Input: part model. Units: mm. Frame: model coordinates. Face numbers are marked on the shaded views. A direction names the side the tool comes from. Coordinates: 2 decimals unless noted, no trailing zeros. Write each loop counter-clockwise with the first axis right and the second up, starting at its lowest first coordinate (ties: lowest second). Pieces come first, ordered by that corner, then holes. Notation, with made-up numbers: (66.25, -38) -> (115.25, -38) arc R10 cw to (115.25, -32) -> close; hole circle Ø6 at (-18, 1). An arc over 180 degrees is marked (long way). Use one line per item in the form item = value. Start each with the question number.
(1) First-contact query: pin 1 (4 mm diameter, centred on x = 6.5, y = -5, fed in from -Z); pin 2 (8.5 mm diameter, centred on x = 7, y = -4, fed in from +Z). Flat tips, straight axial feed; report the tip coordinate or a pass-through.
(2) Cut plane A-A on y = 53.5. Return the cut outline in (x, z).
(3) Cut plane B-B on z = 18. Return the cut outline in (x, y), plus the area to 3 significant figures.
(4) Set-up query: the marked faces 4 and 5. Return all of +Z, -Z, +X, -X, +Y, -Y with unobstructed straight access to the full face (end or side cutting, diameter ignored); none if empty.
(5) Cut plane C-C on x = -27.5. Return the cut outline in (y, z), plus the area to 3 significant figures.
(6) Pull-direction query (Y, two-part tool) for the marked faces 1, 2 and 3; classes: released by +Y, released by -Y, zero draft, split by the parting line, or undercut.
(7) Cut plane D-D on z = 30.5. Return the cut outline in (x, y), plus the area to 3 significant figures.
(8) Ray query, line 1 along X through (y, z) = (20, -16.5); line 2 along Y through (x, z) = (-21.5, -30); line 3 along X through (y, z) = (64, 27.5). Return the intervals inside material, ascending.
```python
from build123d import *

# Parameters (mm, degrees)
SALIENTE_EXTRUIR1_DEPTH = 50
CORTAR_EXTRUIR1_DEPTH   = 10


with BuildPart() as part:
    # Croquis1 → Saliente-Extruir1 (new, symmetric)
    with BuildSketch(Plane.XY):
        Polygon((-50, 0), (50, 0), (50, 60), (20, 60), (20, 67.9375), (57.9375, 67.9375), (57.9375, -7.9375), (-57.9375, -7.9375), (-57.9375, 67.9375), (-20, 67.9375), (-20, 60), (-50, 60), align=None)
    extrude(amount=SALIENTE_EXTRUIR1_DEPTH, both=True)

    # Croquis2 → Cortar-Extruir1 (cut)
    with BuildSketch(Plane.XZ.offset(7.9375)):
        Polygon((-28.867513459, -50), (28.867513459, -50), (14.43375673, -25), (-14.43375673, -25), align=None)
        Polygon((-28.867513459, 50), (28.867513459, 50), (14.43375673, 25), (-14.43375673, 25), align=None)
    extrude(amount=-CORTAR_EXTRUIR1_DEPTH, mode=Mode.SUBTRACT)


solid = part.part
```
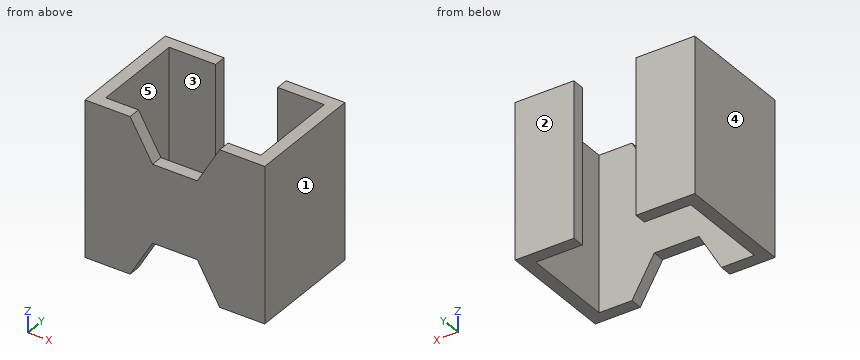
Values:
q1.pin_1 = -25
q1.pin_2 = 25
q2.outline = (-57.94, -50) -> (-50, -50) -> (-50, 50) -> (-57.94, 50) -> close; (50, -50) -> (57.94, -50) -> (57.94, 50) -> (50, 50) -> close
q3.outline = (-57.94, -7.94) -> (57.94, -7.94) -> (57.94, 67.94) -> (20, 67.94) -> (20, 60) -> (50, 60) -> (50, 0) -> (-50, 0) -> (-50, 60) -> (-20, 60) -> (-20, 67.94) -> (-57.94, 67.94) -> close
q3.area = 2,470 mm2
q4.face_4 = +Z, -Z, -X, +Y, -Y
q4.face_5 = +Z, -Z
q5.outline = (-7.94, -47.63) -> (0, -47.63) -> (0, 47.63) -> (-7.94, 47.63) -> close; (60, -50) -> (67.94, -50) -> (67.94, 50) -> (60, 50) -> close
q5.area = 1,550 mm2
q6.face_1 = zero draft
q6.face_2 = released by +Y
q6.face_3 = undercut
q7.outline = (-57.94, -7.94) -> (-17.61, -7.94) -> (-17.61, 0) -> (-50, 0) -> (-50, 60) -> (-20, 60) -> (-20, 67.94) -> (-57.94, 67.94) -> close; (17.61, -7.94) -> (57.94, -7.94) -> (57.94, 67.94) -> (20, 67.94) -> (20, 60) -> (50, 60) -> (50, 0) -> (17.61, 0) -> close
q7.area = 2,190 mm2
q8.line_1 = -57.94 to -50, 50 to 57.94
q8.line_2 = -7.94 to 0, 60 to 67.94
q8.line_3 = -57.94 to -20, 20 to 57.94
